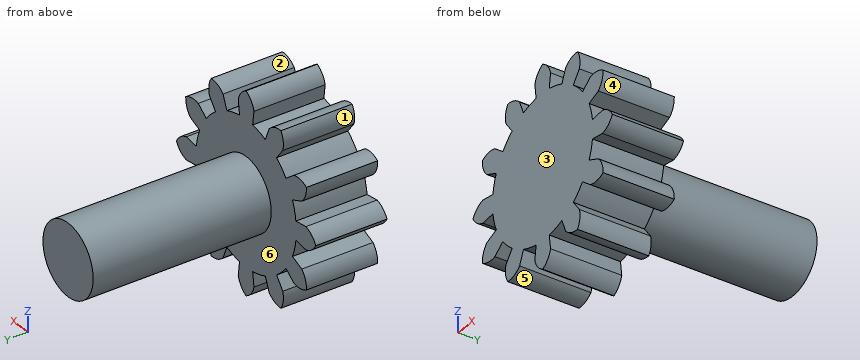
```python
from build123d import *

# Parameters (mm, degrees)
F2_DEPTH        = 10
F2_COPIES_COUNT = 12
F4_R            = 10
F5_DEPTH        = 50


# Not quite as in the source:
# - a feature of the source that left no trace in its solid (it failed there, or was rolled back) is left out
# - a pattern or mirror of a feature is missing from the dataset's text; its kind, count and spacing are read off the source's solid


with BuildPart() as f2:
    # F1 (on Front) → F2 (new body, symmetric)
    with BuildSketch(Plane.XZ):
        with BuildLine():
            ThreePointArc((-2.6105238444, 19.8288972275), (-13.186916302, -15.0367961496), (20, 0))
            ThreePointArc((20, 0), (15.0367961496, 13.186916302), (2.6105238444, 19.8288972275))
            ThreePointArc((2.6105238444, 19.8288972275), (0, 20), (-2.6105238444, 19.8288972275))
        make_face()
        with BuildLine():
            ThreePointArc((-2.6105238444, 19.8288972275), (0, 20), (2.6105238444, 19.8288972275))
            Line((2.6105238444, 19.8288972275), (3.1326286133, 23.794676673))
            ThreePointArc((3.1326286133, 23.794676673), (2.0019466325, 26.1165955987), (0, 27.7481466766))
            ThreePointArc((0, 27.7481466766), (-2.0019466325, 26.1165955987), (-3.1326286133, 23.794676673))
            Line((-3.1326286133, 23.794676673), (-2.6105238444, 19.8288972275))
        make_face()
    extrude(amount=F2_DEPTH, both=True)

    # F2_copies: F2 ×12 about axis
    f2_copies_axis = Axis((0, 0, 0), (0, 1, 0))


with BuildPart() as f2_1:
    add(f2.part)
    for i in range(1, F2_COPIES_COUNT):
        add(f2.part.rotate(f2_copies_axis, i * 360 / F2_COPIES_COUNT))

    # F4 (on face) → F5 (join)
    with BuildSketch(Plane(origin=(0, 10, 0), x_dir=(-1, 0, 0), z_dir=(0, 1, 0))):
        Circle(F4_R)
    extrude(amount=F5_DEPTH)


solid = f2_1.part
```
Source: CAD feature listing. Evaluate the final solid. Frame: model axes, mm. Face numbers are marked on the shaded views. A direction names the side the tool comes from. Give positions to 0.01 mm unless a question says otherwise; leave off trailing zeros. Write each loop counter-clockwise with the first axis right and the second up, starting at its lowest first coordinate (ties: lowest second). Pieces come first, ordered by that corner, then holes.
1. Section query A-A (z = 6.5). Return the cut outline in (x, y), then the cut area to 3 significant figures.
2. Section query B-B (y = 46). Return the cut outline in (x, z).
3. Pull-direction query (Z, two-part tool) for the marked faces 1, 2 and 3; classes: +Z half, -Z half, draft (parallel to the pull), parting line (faces both ways), or undercut.
4. Section query C-C (x = 11). Return the cut outline in (y, z).
5. Access query for the marked faces 4, 5 and 6. Directions: +Z, -Z, +X, -X, +Y, -Y. A direction counts if a zero-diameter tool reaches every point of the face in a straight line with its end or side. Return the directions, or none.
6. First-contact query: pin 1 (5 mm diameter, centred on x = -21, y = 10.5, fed in from +Z); pin 2 (12 mm diameter, centred on x = -3.5, y = 39.5, fed in from +Z). Flat tips, straight axial feed; report the tip coordinate or a pass-through.
7. Material intervals for line 1 along Z through (x, y) = (-23, -3); line 2 along Y through (x, z) = (-0.5, 19.5); line 3 along X through (y, z) = (55, 3), sorted ascending.
Output values:
1. outline: (-18.91, -10) - (18.91, -10) - (18.91, 10) - (7.6, 10) - (7.6, 60) - (-7.6, 60) - (-7.6, 10) - (-18.91, 10) - close
1. area: 1,520 mm2
2. outline: circle Ø20 at (0, 0)
3. face 1: undercut
3. face 2: +Z half
3. face 3: draft
4. outline: (-10, -23.48) - (10, -23.48) - (10, 23.48) - (-10, 23.48) - close
5. face 4: +X, +Y, -Y
5. face 5: -Z, +Y, -Y
5. face 6: +Y
6. pin 1: stops at z = 14.86
6. pin 2: stops at z = 10
7. line 1: z = -14.41 to -10.16, -3.03 to 3.03, 10.16 to 14.41
7. line 2: y = -10 to 10
7. line 3: x = -9.54 to 9.54
